Could you check a few things on this drawing? It's one solid part, dimensions in mm from its lowest x, y, z. Give positions to 0.01 mm unless a question says otherwise; leave off trailing zeros. Write each loop counter-clockwise with the first axis right and the second up, starting at its lowest first coordinate (ties: lowest second). Pieces come first, ordered by that corner, then holes. Notation, with made-up numbers: (68, 55.5) -> (100, 55.5) arc R31 cw to (100, 83.5) -> close; hole circle Ø4 at (59.25, 81). An arc over 180 degrees is marked (long way). Use CSV: the item, a comma, the result in double quotes. Start each with the question number.
(1) I need wall thicknesses on L1, parallel to X at y = 54, z = 3; L2, parallel to X at y = 79.5, z = 5.5; L3, parallel to Y at x = 12, z = 13.75 (1 decimal). Which ranges of each line are inside material? Lowest first, please. Write a range as [from, to].
(2) For pin 1 Ø5 at (y, z) = (64, 13) entering from -X; pin 2 Ø1.5 at (x, z) = (14.5, 8) entering from +Y (1 decimal); pin 3 Ø4 at (x, y) = (55, 68.5) entering from -Z, each with a flat end and sliding along its axis, tell me the tip position at first contact or that it passes through.
(3) Suppose I cut it at B-B on y = 44.5. List the corners of the cut face in (x, z) for me (1 decimal).
(4) Suppose I cut it at C-C on y = 79. List the corners of the cut face in (x, z) for me, plus the area to 3 significant figures.
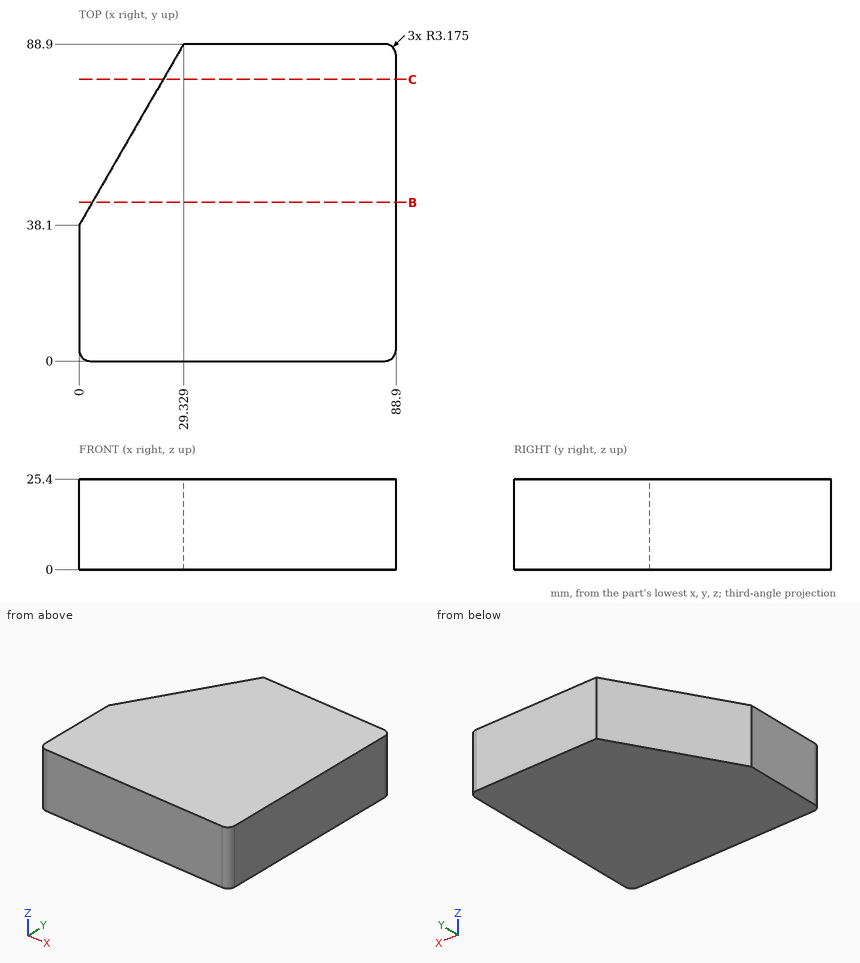
Geometry says:
1,L1,"[9.18, 88.9]"
1,L2,"[23.9, 88.9]"
1,L3,"[0, 58.9]"
2,pin 1,"x = 13.51"
2,pin 2,"y = 64.5"
2,pin 3,"z = 0"
3,outline,"(3.7, 0) -> (88.9, 0) -> (88.9, 25.4) -> (3.7, 25.4) -> close"
4,outline,"(23.61, 0) -> (88.9, 0) -> (88.9, 25.4) -> (23.61, 25.4) -> close"
4,area,"1,660 mm²"
